```python
from build123d import *

# Parameters (mm, degrees)
EXTRUDE_1_DEPTH     = 10
SKETCH_4_R          = 2.25
CUT_EXTRUDE_1_DEPTH = 10
SKETCH_2_R          = 2.25
CUT_EXTRUDE_2_DEPTH = 27
FILLET_2_R          = 0.5
FILLET_3_R          = 1
FILLET_4_R          = 4


with BuildPart() as part:
    # 草图1 → 凸台-拉伸1 (new body)
    with BuildSketch(Plane.XY):
        with BuildLine():
            Line((-8, 0), (-8, -17))
            ThreePointArc((-8, -17), (-8.585786438, -18.414213562), (-10, -19))
            Line((-10, -19), (-10.5, -19))
            ThreePointArc((-10.5, -19), (-10.853553391, -18.853553391), (-11, -18.5))
            Line((-11, -18.5), (-11, 3))
            Line((-11, 3), (11, 3))
            Line((11, 3), (11, -18.5))
            ThreePointArc((11, -18.5), (10.853553391, -18.853553391), (10.5, -19))
            Line((10.5, -19), (10, -19))
            ThreePointArc((10, -19), (8.585786438, -18.414213562), (8, -17))
            Line((8, -17), (8, 0))
            Line((8, 0), (-8, 0))
        make_face()
    extrude(amount=EXTRUDE_1_DEPTH)

    # 草图4 → 切除-拉伸1 (cut)
    with BuildSketch(Plane(origin=(0, 0, 0), x_dir=(1, 0, 0), z_dir=(0, 1, 0))):
        with Locations((0, -5)):
            Circle(SKETCH_4_R)
    extrude(amount=CUT_EXTRUDE_1_DEPTH, mode=Mode.SUBTRACT)

    # 草图2 → 切除-拉伸2 (cut)
    with BuildSketch(Plane(origin=(11, 0, 0), x_dir=(0, 0, -1), z_dir=(1, 0, 0))):
        with Locations((-5, -8)):
            Circle(SKETCH_2_R)
    extrude(amount=-CUT_EXTRUDE_2_DEPTH, mode=Mode.SUBTRACT)

    # 圆角2
    fillet_2_edges = [part.edges().sort_by_distance(p)[0] for p in [
        (-2.25, 0, 5),
        (-8, -8, 7.25),
        (8, -8, 7.25),
    ]]
    fillet(fillet_2_edges, radius=FILLET_2_R)

    # 圆角3
    fillet_3_edges = [part.edges().sort_by_distance(p)[0] for p in [
        (-11, 3, 5),
        (11, 3, 5),
    ]]
    fillet(fillet_3_edges, radius=FILLET_3_R)

    # 圆角4
    fillet_4_edges = [part.edges().sort_by_distance(p)[0] for p in [
        (8, 0, 5),
        (-8, 0, 5),
    ]]
    fillet(fillet_4_edges, radius=FILLET_4_R)


solid = part.part
```
Work out the finished part from the listing and answer in its coordinate system (mm). A direction names the side the tool comes from. Coordinates: 2 decimals unless noted, no trailing zeros. Write each loop counter-clockwise with the first axis right and the second up, starting at its lowest first coordinate (ties: lowest second). Pieces come first, ordered by that corner, then holes. Notation, with made-up numbers: (6, 3) - (37, 3) arc R30 ccw to (37, 33) - close; hole circle Ø2 at (-3.5, 6.25). An arc over 180 degrees is marked (long way). Answer as a JSON object with one key per item and string values.
Q1. Find section B-B (z = 5). State how many separate pieces and enclosed holes the cut face has, plus the area to 3 significant figures.
Results list:
{"separate pieces": "4", "enclosed holes": "0", "area": "144 mm^2"}
Q2. For a pull along Z with two mould halves and no side action, classify faces 3 (the cylindrical face through (-0.488, 1.732, 7.196)), 4 (the cylindrical face through (-8.57, -18.4, 4.93)), 5 (the flat face through (0.9, 0.2, 10)) as pulls with the +Z half, pulls with the -Z half, needs draft (parallel to the pull), parting line crosses it, or undercut.
Results list:
{"face 3": "undercut", "face 4": "needs draft", "face 5": "pulls with the +Z half"}
Q3. Given pin 1 Ø3 at (x, z) = (7.5, 4) entering from -Y; pin 2 Ø4 at (x, z) = (-0.5, 7.5) entering from -Y; pin 3 Ø4 at (x, y) = (-4.5, -6) entering from -Z, each flat-ended and moving along its own axis, determine where each tip first touches the part or whether it passes through.
Results list:
{"pin 1": "stops at y = -18.73", "pin 2": "stops at y = 0", "pin 3": "passes through"}
Q4. Find section C-C (y = -8). Write down the section's boundary in (x, z), plus the area to 3 significant figures.
Results list:
{"outline": "(-11, 0) - (-8, 0) - (-8, 2.25) arc R0.5 ccw to (-8.5, 2.75) - (-11, 2.75) - close; (-11, 7.25) - (-8.5, 7.25) arc R0.5 ccw to (-8, 7.75) - (-8, 10) - (-11, 10) - close; (8, 0) - (11, 0) - (11, 2.75) - (8.5, 2.75) arc R0.5 ccw to (8, 2.25) - close; (8, 7.75) arc R0.5 ccw to (8.5, 7.25) - (11, 7.25) - (11, 10) - (8, 10) - close", "area": "32.8 mm^2"}
Q5. Find section A-A (x = 0). Write down the section's boundary in (y, z), plus the area to 3 significant figures.
Results list:
{"outline": "(0, 0) - (3, 0) - (3, 2.75) - (0.5, 2.75) arc R0.5 ccw to (0, 2.25) - close; (0, 7.75) arc R0.5 ccw to (0.5, 7.25) - (3, 7.25) - (3, 10) - (0, 10) - close", "area": "16.4 mm^2"}
Q6. Consider L1, parallel to X at y = -5.25, z = 3.5; L2, parallel to Z at x = 0, y = 1; L3, parallel to Y at x = 10.05, z = 5. Determine where each line is inside the solid, lowest interval first. Write a range as from..to.
Results list:
{"L1": "x = -11..-8, 8..11", "L2": "z = 0..2.75, 7.25..10", "L3": "y = -19..-10.25, -5.75..3"}
Q7. Which of the six approach directions +Z, -Z, +X, -X, +Y, -Y give full straight-line access (tool end or side, diameter ignored) to faces 1 (the flat face through (-11, -11, 5)), 2 (the cylindrical face through (-6.859, -1.203, 5.07))?
Results list:
{"face 1": "+Z, -Z, -X, +Y, -Y", "face 2": "+Z, -Z, -Y"}
Q8. Find section D-D (z = 9). Write down the section's boundary in (x, y), plus the area to 3 significant figures.
Results list:
{"outline": "(-11, -18.5) arc R0.5 ccw to (-10.5, -19) - (-10, -19) arc R2 ccw to (-8, -17) - (-8, -4) arc R4 cw to (-4, 0) - (4, 0) arc R4 cw to (8, -4) - (8, -17) arc R2 ccw to (10, -19) - (10.5, -19) arc R0.5 ccw to (11, -18.5) - (11, 2) arc R1 ccw to (10, 3) - (-10, 3) arc R1 ccw to (-11, 2) - close", "area": "185 mm^2"}
